from build123d import *

# Parameters (mm, degrees)
BOSS_EXTRUDE1_START = -12.7
BOSS_EXTRUDE1_DEPTH = 12.7
BOSS_EXTRUDE2_START = -63.5
BOSS_EXTRUDE2_DEPTH = 25.4


with BuildPart() as part:
    # Sketch1 → Revolve1 (revolve)
    with BuildSketch(Plane.XY, mode=Mode.PRIVATE) as revolve1_sk:
        Polygon((0, 9.525), (64.643, 9.525), (64.643, 5.1435), (74.168, 5.1435), (74.168, 1.5875), (59.77878359, 1.5875), (59.77878359, 4.58916283), (40.457949701, 4.58916283), (40.457949701, 7.536935058), (36.795436007, 7.536935058), (36.795436007, 5.555870047), (31.917498279, 2.413), (25.308223812, 2.413), (23.794433849, 4.7625), (0, 4.7625), align=None)
    revolve(revolve1_sk.sketch.rotate(Axis((0, 0, 0), (1, 0, 0)), 90), axis=Axis((0, 0, 0), (1, 0, 0)))

    # Sketch8 → Boss-Extrude1 (add)
    with BuildSketch(Plane.ZY.offset(BOSS_EXTRUDE1_START)):
        with BuildLine():
            Line((5.499261314, 9.525), (0, 9.525))
            ThreePointArc((0, 9.525), (4.762499953, 8.248891998), (8.248891917, 4.762500094))
            Line((8.248891917, 4.762500094), (5.499261314, 9.525))
        make_face()
        with BuildLine():
            Line((-5.499261314, 9.525), (-8.248892028, 4.762499902))
            ThreePointArc((-8.248892028, 4.762499902), (-4.762500049, 8.248891943), (0, 9.525))
            Line((0, 9.525), (-5.499261314, 9.525))
        make_face()
        with BuildLine():
            Line((-8.248892028, 4.762499902), (-10.998522628, 0))
            Line((-10.998522628, 0), (-8.248891917, -4.762500094))
            ThreePointArc((-8.248891917, -4.762500094), (-9.525, -1.11e-07), (-8.248892028, 4.762499902))
        make_face()
        with BuildLine():
            ThreePointArc((0, -9.525), (-4.762499953, -8.248891998), (-8.248891917, -4.762500094))
            Line((-8.248891917, -4.762500094), (-5.499261314, -9.525))
            Line((-5.499261314, -9.525), (0, -9.525))
        make_face()
        with BuildLine():
            ThreePointArc((8.248891846, -4.762500216), (4.762499892, -8.248892033), (0, -9.525))
            Line((0, -9.525), (5.499261314, -9.525))
            Line((5.499261314, -9.525), (8.248891846, -4.762500216))
        make_face()
        with BuildLine():
            ThreePointArc((9.525, 0), (9.200443463, -2.465251525), (8.248891846, -4.762500216))
            Line((8.248891846, -4.762500216), (10.998522628, 0))
            Line((10.998522628, 0), (8.248891917, 4.762500094))
            ThreePointArc((8.248891917, 4.762500094), (9.200443481, 2.465251457), (9.525, 0))
        make_face()
    extrude(amount=BOSS_EXTRUDE1_DEPTH)

    # Sketch8_3 → Boss-Extrude2 (add)
    with BuildSketch(Plane.ZY.offset(BOSS_EXTRUDE2_START)):
        with BuildLine():
            Line((5.499261314, 9.525), (0, 9.525))
            ThreePointArc((0, 9.525), (4.762499953, 8.248891998), (8.248891917, 4.762500094))
            Line((8.248891917, 4.762500094), (5.499261314, 9.525))
        make_face()
        with BuildLine():
            Line((-5.499261314, 9.525), (-8.248892028, 4.762499902))
            ThreePointArc((-8.248892028, 4.762499902), (-4.762500049, 8.248891943), (0, 9.525))
            Line((0, 9.525), (-5.499261314, 9.525))
        make_face()
        with BuildLine():
            Line((-8.248892028, 4.762499902), (-10.998522628, 0))
            Line((-10.998522628, 0), (-8.248891917, -4.762500094))
            ThreePointArc((-8.248891917, -4.762500094), (-9.525, -1.11e-07), (-8.248892028, 4.762499902))
        make_face()
        with BuildLine():
            ThreePointArc((0, -9.525), (-4.762499953, -8.248891998), (-8.248891917, -4.762500094))
            Line((-8.248891917, -4.762500094), (-5.499261314, -9.525))
            Line((-5.499261314, -9.525), (0, -9.525))
        make_face()
        with BuildLine():
            ThreePointArc((8.248891846, -4.762500216), (4.762499892, -8.248892033), (0, -9.525))
            Line((0, -9.525), (5.499261314, -9.525))
            Line((5.499261314, -9.525), (8.248891846, -4.762500216))
        make_face()
        with BuildLine():
            ThreePointArc((9.525, 0), (9.200443463, -2.465251525), (8.248891846, -4.762500216))
            Line((8.248891846, -4.762500216), (10.998522628, 0))
            Line((10.998522628, 0), (8.248891917, 4.762500094))
            ThreePointArc((8.248891917, 4.762500094), (9.200443481, 2.465251457), (9.525, 0))
        make_face()
    extrude(amount=BOSS_EXTRUDE2_DEPTH)


solid = part.part
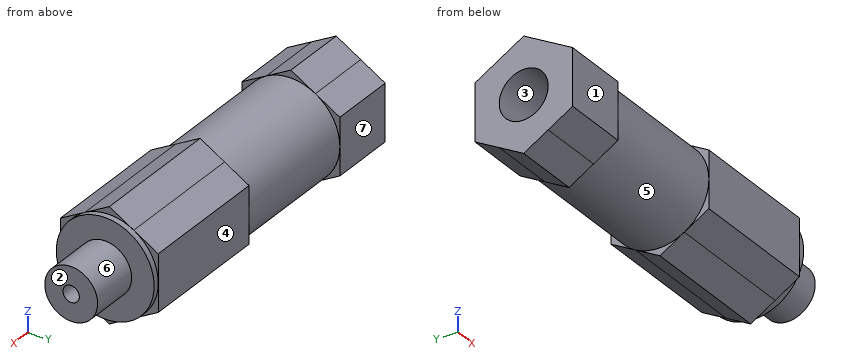
Geometry check sheet. Reference: the model listing, model coordinates, mm. Face numbers are marked on the shaded views. A direction names the side the tool comes from. Round coordinates to 2 decimals unless told otherwise and drop trailing zeros. Order: outer loops, then holes, each group sorted by start corner. A loop starts at its lowest first (then second) coordinate and runs counter-clockwise, first axis right, second up. Notation, with made-up numbers: M 26.5,84 L 72.5,84 A23 cw 72.5,109 Z; hole C 17.5,-19 d2. An arc over 180 degrees is marked long. Answer in a Markdown table with one row per item. Add a question column.
Item 1: Sectioned sample at B-B, the plane z = 6.25. Enter the section's corners in (x, y).
Item 2: Material ranges on L1, parallel to Y at x = 6.5, z = 0 (1 decimal); L2, parallel to Y at x = 70, z = 0; L3, parallel to X at y = 6.75, z = 0, recorded low to high. Write a range as [from, to].
Item 3: Sectioned sample at D-D, the plane x = 35. Enter the section's corners in (y, z) (3 decimals).
Item 4: Draft check along Y on the marked faces 1, 2, 3 and 4. Enter one of: released by +Y, released by -Y, zero draft, split by the parting line, or undercut.
Item 5: Sectioned sample at C-C, the plane x = 43. Enter the section's corners in (y, z) (1 decimal), plus the area to 3 significant figures.
Item 6: Set-up check for the marked faces 5, 6 and 7: record each of +Z, -Z, +X, -X, +Y, -Y from which the full face is reachable in a straight line by a thin tool's end or side.
Item 7: Depth check by flat-ended pin: pin 1 Ø4 at (y, z) = (6.5, -2.5) entering from +X; pin 2 Ø5 at (y, z) = (2, -7.5) entering from +X; pin 3 Ø6 at (x, y) = (65, 7) entering from +Z; pin 4 Ø5 at (x, y) = (28.5, 7.5) entering from +Z. Enter the tip coordinate at first touch or a pass-through.
Item 8: Sectioned sample at A-A, the plane x = 8. Enter the section's corners in (y, z) (1 decimal).
Filled in:
| question | item | result |
|---|---|---|
| 1 | outline | M 0,-8.22 L 12.7,-8.22 L 12.7,-7.19 L 38.1,-7.19 L 38.1,-8.22 L 63.5,-8.22 L 63.5,-7.19 L 64.64,-7.19 L 64.64,7.19 L 63.5,7.19 L 63.5,8.22 L 38.1,8.22 L 38.1,7.19 L 12.7,7.19 L 12.7,8.22 L 0,8.22 Z; hole M 36.8,-4.21 L 40.46,-4.21 L 40.46,4.21 L 36.8,4.21 Z |
| 2 | L1 | y = [-9.5, -4.8], [4.8, 9.5] |
| 2 | L2 | y = [-5.14, -1.59], [1.59, 5.14] |
| 2 | L3 | x = [0, 36.8], [40.46, 64.64] |
| 3 | outline | C 0,0 d19.05; hole C 0,0 d8.798 |
| 4 | face 1 | released by -Y |
| 4 | face 2 | zero draft |
| 4 | face 3 | undercut |
| 4 | face 4 | released by +Y |
| 5 | outline | M -9.5,-5.5 L 0,-11 L 9.5,-5.5 L 9.5,5.5 L 0,11 L -9.5,5.5 Z; hole C 0,0 d9.2 |
| 5 | area | 248 mm² |
| 6 | face 5 | none |
| 6 | face 6 | +X |
| 6 | face 7 | +Z, -Z, +X, -X, +Y |
| 7 | pin 1 | stops at x = 74.17 |
| 7 | pin 2 | stops at x = 64.64 |
| 7 | pin 3 | stops at z = 8.63 |
| 7 | pin 4 | stops at z = 8.11 |
| 8 | outline | M -9.5,-5.5 L 0,-11 L 9.5,-5.5 L 9.5,5.5 L 0,11 L -9.5,5.5 Z; hole C 0,0 d9.5 |
